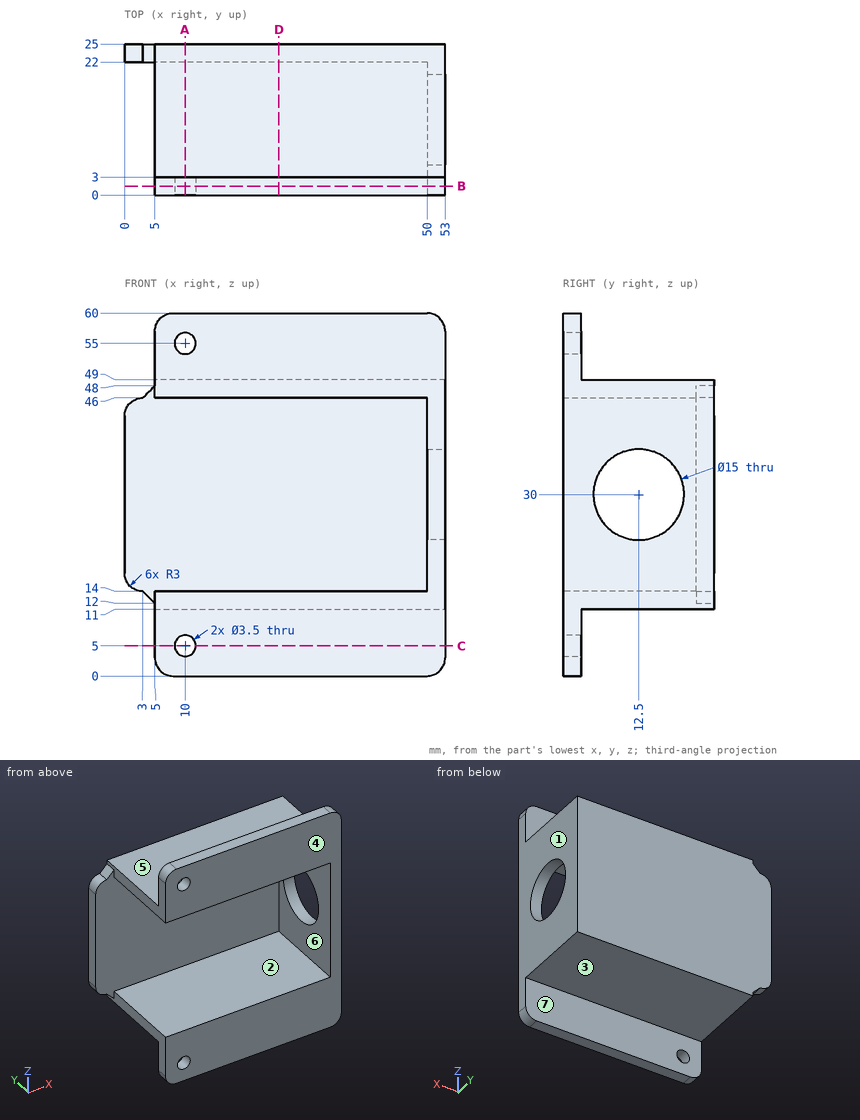
Here's the drawing with two shaded views (mm, measured from the low corner). I have some questions. A direction names the side the tool comes from. Give positions to 0.01 mm unless a question says otherwise; leave off trailing zeros. Loops run counter-clockwise (first coordinate to the right, second up) from the corner with the lowest first, then second, coordinate; pieces in that order, holes last. Notation, with made-up numbers: M 73.25,84.25 L 86.25,84.25 A13 cw 86.25,106.25 Z; hole C 71.25,54 d7. An arc over 180 degrees is marked long. One line per item, written item: value. Start each with the question number.
1) If we section it at D-D, the plane x = 25.5: Write out the boundary of the cut face in (y, z), and give its area (3 significant figures).
2) Thinking about a two-plate mould opening in Z: for the marked faces 1, 2 and 3, which applies, +Z half, -Z half, draft (parallel to the pull), parting line (faces both ways), or undercut?
3) If we section it at A-A, the plane x = 10: Write out the boundary of the cut face in (y, z).
4) If we section it at B-B, the plane y = 1.5: Write out the boundary of the cut face in (x, z).
5) If I drill on line 1 (Z direction, x = 43, y = 5); line 2 (X direction, y = 1, z = 55); line 3 (Z direction, x = 43, y = 1.5), over which ranges is the centre line in solid material (lowest first)? Write a range as [from, to].
6) On a 3-axis mill with a long thin cutter (end or side, diameter ignored), from which of +Z, -Z, +X, -X, +Y, -Y can I reach the whole of each face in a straight line? I mean the marked faces 4, 5, 6 and 7. Say none if no direction works.
7) If we section it at C-C, the plane z = 5: Write out the boundary of the cut face in (x, y), and give its area (4 significant figures).
8) I'm going to push flat-ended pins straight in: pin 1 (9 mm diameter, centred on y = 11, z = 11, fed in from -X); pin 2 (3 mm diameter, centred on y = 8.5, z = 41.5, fed in from -X); pin 3 (5.5 mm diameter, centred on x = 33.5, z = 4, fed in from +Y); pin 4 (3 mm diameter, centred on x = 10, z = 55, fed in from -Y). Where does each tip first touch, or does it pass through?
Completed:
1. outline: M 0,0 L 3,0 L 3,11 L 25,11 L 25,49 L 3,49 L 3,60 L 0,60 L 0,46 L 22,46 L 22,14 L 0,14 Z
1. area: 312 mm^2
2. face 1: draft
2. face 2: undercut
2. face 3: -Z half
3. outline: M 0,0 L 3,0 L 3,3.25 L 0,3.25 Z; M 0,6.75 L 3,6.75 L 3,11 L 25,11 L 25,49 L 3,49 L 3,53.25 L 0,53.25 L 0,46 L 22,46 L 22,14 L 0,14 Z; M 0,56.75 L 3,56.75 L 3,60 L 0,60 Z
4. outline: M 5,3 A3 ccw 8,0 L 50,0 A3 ccw 53,3 L 53,57 A3 ccw 50,60 L 8,60 A3 ccw 5,57 L 5,46 L 50,46 L 50,14 L 5,14 Z; hole C 10,5 d3.5; hole C 10,55 d3.5
5. line 1: z = [11, 14], [46, 49]
5. line 2: x = [5, 8.25], [11.75, 53]
5. line 3: z = [0, 14], [46, 60]
6. face 4: +Z, -Z, +X, -X, -Y
6. face 5: +Z, +X, -X, +Y
6. face 6: -X, -Y
6. face 7: -Z, +X, -X, +Y
7. outline: M 5,0 L 8.25,0 L 8.25,3 L 5,3 Z; M 11.75,0 L 53,0 L 53,3 L 11.75,3 Z
7. area: 133.5 mm^2
8. pin 1: stops at x = 5
8. pin 2: stops at x = 50
8. pin 3: stops at y = 3
8. pin 4: passes through
